from build123d import *

# Parameters (mm, degrees)
BOSS_EXTRUDE1_DEPTH  = 3.5
BOSS_EXTRUDE2_DEPTH  = 21
SKETCH3_W            = 23
SKETCH3_H            = 39
BOSS_EXTRUDE3_DEPTH  = 2.5
SKETCH5_W            = 21.5
SKETCH5_H            = 25
SKETCH5_W_2          = 7.07
SKETCH5_H_2          = 19.04
BOSS_EXTRUDE5_DEPTH  = 2.5
SKETCH6_W            = 7.07
SKETCH6_H            = 5.9
BOSS_EXTRUDE6_DEPTH  = 20
BOSS_EXTRUDE7_DEPTH  = 23
FILLET1_SIZE         = 10
SKETCH9_R            = 2.475
BOSS_EXTRUDE8_DEPTH  = 9
FILLET2_R            = 0.5
SKETCH10_R           = 1.65
CUT_EXTRUDE1_DEPTH   = 9
SKETCH11_W           = 0.2
SKETCH11_H           = 20
CUT_EXTRUDE2_DEPTH   = 9
CUT_EXTRUDE3_DEPTH   = 9
FILLET3_SIZE         = 3
BOSS_EXTRUDE9_DEPTH  = 5
SKETCH14_R           = 1.747814763
SKETCH14_R_2         = 1.6
CUT_EXTRUDE4_DEPTH   = 15
SKETCH15_W           = 110
SKETCH15_H           = 3.5
CUT_EXTRUDE5_DEPTH   = 150
FILLET4_SIZE         = 7
FILLET5_SIZE         = 3
FILLET6_SIZE         = 3
SKETCH17_W           = 8
SKETCH17_H           = 21
CUT_EXTRUDE6_DEPTH   = 150
FILLET7_R            = 1
FILLET9_SIZE         = 3
SKETCH19_R           = 1.747814763
SKETCH19_R_2         = 1.6
BOSS_EXTRUDE10_DEPTH = 8.43
CUT_EXTRUDE7_DEPTH   = 8.43
FILLET10_R           = 1


# Some blends are built 0.0001 mm under size
with BuildPart() as part:
    # Sketch1 → Boss-Extrude1 (new body)
    with BuildSketch(Plane(origin=(0, 0, 0), x_dir=(1, 0, 0), z_dir=(0, 1, 0))):
        Polygon((0, 40), (23, 40), (23, 79), (0, 79), (0, 100), (110, 100), (110, 79), (87, 79), (87, 40), (110, 40), (110, 20), (80, 0), (30, 0), (0, 20), align=None)
    extrude(amount=BOSS_EXTRUDE1_DEPTH)

    # Sketch2 → Boss-Extrude2 (add)
    with BuildSketch(Plane(origin=(0, 3.5, 0), x_dir=(1, 0, 0), z_dir=(0, 1, 0))):
        Polygon((0, 79), (23, 79), (23, 40), (0, 40), (0, 37.5), (25.5, 37.5), (25.5, 81.5), (0, 81.5), align=None)
        Polygon((110, 81.5), (84.5, 81.5), (84.5, 37.5), (110, 37.5), (110, 40), (87, 40), (87, 79), (110, 79), align=None)
    extrude(amount=BOSS_EXTRUDE2_DEPTH)

    # Sketch3 → Boss-Extrude3 (add)
    with BuildSketch(Plane(origin=(0, 24.5, 0), x_dir=(1, 0, 0), z_dir=(0, 1, 0))):
        with Locations((11.5, 59.5)):
            Rectangle(SKETCH3_W, SKETCH3_H)
        with Locations((98.5, 59.5)):
            Rectangle(SKETCH3_W, SKETCH3_H)
    extrude(amount=-BOSS_EXTRUDE3_DEPTH)

    # Sketch5 → Boss-Extrude5 (add)
    with BuildSketch(Plane(origin=(0, 24.5, 0), x_dir=(1, 0, 0), z_dir=(0, 1, 0))):
        with Locations((120.75, 50)):
            Rectangle(SKETCH5_W, SKETCH5_H)
        with Locations((-10.75, 50)):
            Rectangle(SKETCH5_W, SKETCH5_H)
        with Locations((29.035, 47.02)):
            Rectangle(SKETCH5_W_2, SKETCH5_H_2)
        with Locations((80.965, 47.02)):
            Rectangle(SKETCH5_W_2, SKETCH5_H_2)
    extrude(amount=-BOSS_EXTRUDE5_DEPTH)

    # Sketch6 → Boss-Extrude6 (add)
    with BuildSketch(Plane(origin=(0, 24.5, 0), x_dir=(1, 0, 0), z_dir=(0, 1, 0))):
        with Locations((29.035, 53.59)):
            Rectangle(SKETCH6_W, SKETCH6_H)
        with Locations((80.965, 53.59)):
            Rectangle(SKETCH6_W, SKETCH6_H)
        with Locations((-17.965, 53.59)):
            Rectangle(SKETCH6_W, SKETCH6_H)
        with Locations((127.965, 53.59)):
            Rectangle(SKETCH6_W, SKETCH6_H)
    extrude(amount=BOSS_EXTRUDE6_DEPTH)

    # Sketch7 → Boss-Extrude7 (add)
    with BuildSketch(Plane(origin=(0, 24.5, 0), x_dir=(1, 0, 0), z_dir=(0, 1, 0))):
        Polygon((0, 81.5), (25.5, 81.5), (25.5, 79), (0, 79), (-21.5, 79), (-21.5, 81.5), align=None)
        Polygon((110, 79), (84.5, 79), (84.5, 81.5), (110, 81.5), (131.5, 81.5), (131.5, 79), align=None)
    extrude(amount=BOSS_EXTRUDE7_DEPTH)

    # Fillet1
    # the kernel refuses this chamfer: 10 mm, written as the material it adds along each edge
    with BuildSketch(Plane(origin=(0, 22, -40), x_dir=(0.027495876610586372, -0.9996219169112968, 0), z_dir=(0, 0, 1)), Plane(origin=(110, 22, -37.5), x_dir=(-0.027495876610586317, -0.9996219169112968, 0), z_dir=(0, 0, -1)), Plane(origin=(110, 24.5, -81.5), x_dir=(0.9996219169112968, 0.027495876610586317, 0), z_dir=(0, 0, 1))) as fillet1_piece_1:
        Polygon((FILLET1_SIZE * 0.999621916911, -FILLET1_SIZE * 0.0274958766106), (-FILLET1_SIZE * 0.0274958766106, -FILLET1_SIZE * 0.999621916911), (0, 0), align=None)
    extrude(amount=2.5)
    with BuildSketch(Plane(origin=(0, 24.5, -79), x_dir=(0.027495876610586372, -0.9996219169112968, 0), z_dir=(0, 0, -1))) as fillet1_piece_2:
        Polygon((FILLET1_SIZE * 0.999621916911, FILLET1_SIZE * 0.0274958766106), (-FILLET1_SIZE * 0.0274958766106, FILLET1_SIZE * 0.999621916911), (0, 0), align=None)
    extrude(amount=2.5)

    # Sketch9 → Boss-Extrude8 (add)
    with BuildSketch(Plane(origin=(0, 0, -81.5), x_dir=(-1, 0, 0), z_dir=(0, 0, -1))):
        with Locations(Location((-114.55, 34.35, 0), (0, 0, 180))):
            Circle(SKETCH9_R)
        with Locations(Location((4.55, 34.35, 0), (0, 0, 180))):
            Circle(SKETCH9_R)
    extrude(amount=BOSS_EXTRUDE8_DEPTH)

    # Fillet2
    fillet2_edges = [part.edges().sort_by_distance(p)[0] for p in [
        (112.075, 34.35, -90.5),
        (-7.025, 34.35, -90.5),
    ]]
    fillet(fillet2_edges, radius=FILLET2_R)

    # Sketch10 → Cut-Extrude1 (cut)
    with BuildSketch(Plane.XY.offset(-50.64)):
        with Locations((129.16, 39.27)):
            Circle(SKETCH10_R)
        with Locations((129.16, 29.43)):
            Circle(SKETCH10_R)
        with Locations((79.77, 39.27)):
            Circle(SKETCH10_R)
        with Locations((79.77, 29.43)):
            Circle(SKETCH10_R)
        with Locations((-19.16, 29.43)):
            Circle(SKETCH10_R)
        with Locations((-19.16, 39.27)):
            Circle(SKETCH10_R)
        with Locations(Location((30.23, 39.27, 0), (0, 0, 180))):
            Circle(SKETCH10_R)
        with Locations(Location((30.23, 29.43, 0), (0, 0, 180))):
            Circle(SKETCH10_R)
    extrude(amount=-CUT_EXTRUDE1_DEPTH, mode=Mode.SUBTRACT)

    # Sketch11 → Cut-Extrude2 (cut)
    with BuildSketch(Plane.XY.offset(-50.64)):
        with Locations((-14.53, 34.5)):
            Rectangle(SKETCH11_W, SKETCH11_H)
        with Locations((25.6, 34.5)):
            Rectangle(SKETCH11_W, SKETCH11_H)
        with Locations((84.4, 34.5)):
            Rectangle(SKETCH11_W, SKETCH11_H)
        with Locations((124.53, 34.5)):
            Rectangle(SKETCH11_W, SKETCH11_H)
    extrude(amount=-CUT_EXTRUDE2_DEPTH, mode=Mode.SUBTRACT)

    # Sketch12 → Cut-Extrude3 (cut)
    with BuildSketch(Plane(origin=(0, 0, -81.5), x_dir=(-1, 0, 0), z_dir=(0, 0, -1))):
        Polygon((-108, 47.5), (-84.5, 25.5), (-84.5, 47.5), align=None)
        Polygon((-25.5, 25.5), (-25.5, 47.5), (-2, 47.5), align=None)
        Polygon((-120, 24.5), (-131.5, 36), (-131.5, 24.5), align=None)
        Polygon((10, 24.5), (21.5, 36), (21.5, 24.5), align=None)
    extrude(amount=-CUT_EXTRUDE3_DEPTH, mode=Mode.SUBTRACT)

    # Fillet3
    fillet3_edges = [part.edges().sort_by_distance(p)[0] for p in [
        (0, 23.25, -62.5),
        (110, 23.25, -62.5),
    ]]
    chamfer(fillet3_edges, length=FILLET3_SIZE)

    # Sketch13 → Boss-Extrude9 (add)
    with BuildSketch(Plane(origin=(0, 3.5, 0), x_dir=(1, 0, 0), z_dir=(0, 1, 0))):
        Polygon((0, 30.5), (32.5, 30.5), (32.5, 88.5), (0, 88.5), (0, 81.5), (25.5, 81.5), (25.5, 37.5), (0, 37.5), align=None)
        Polygon((84.5, 37.5), (110, 37.5), (110, 30.5), (77.5, 30.5), (77.5, 88.5), (110, 88.5), (110, 81.5), (84.5, 81.5), align=None)
    extrude(amount=BOSS_EXTRUDE9_DEPTH)

    # Sketch14 → Cut-Extrude4 (cut)
    with BuildSketch(Plane(origin=(0, 8.5, 0), x_dir=(1, 0, 0), z_dir=(0, 1, 0))):
        with Locations(Location((7.25, 34, 0), (0, 0, 270))):
            Circle(SKETCH14_R)
        with Locations(Location((7.25, 85, 0), (0, 0, 270))):
            Circle(SKETCH14_R_2)
        with Locations(Location((29, 34, 0), (0, 0, 270))):
            Circle(SKETCH14_R_2)
        with Locations(Location((29, 59.5, 0), (0, 0, 270))):
            Circle(SKETCH14_R_2)
        with Locations(Location((29, 85, 0), (0, 0, 270))):
            Circle(SKETCH14_R_2)
        with Locations(Location((81, 34, 0), (0, 0, 90))):
            Circle(SKETCH14_R_2)
        with Locations(Location((102.75, 34, 0), (0, 0, 90))):
            Circle(SKETCH14_R)
        with Locations(Location((81, 59.5, 0), (0, 0, 90))):
            Circle(SKETCH14_R_2)
        with Locations(Location((81, 85, 0), (0, 0, 90))):
            Circle(SKETCH14_R_2)
        with Locations(Location((102.75, 85, 0), (0, 0, 90))):
            Circle(SKETCH14_R_2)
    extrude(amount=-CUT_EXTRUDE4_DEPTH, mode=Mode.SUBTRACT)

    # Sketch15 → Cut-Extrude5 (cut)
    with BuildSketch(Plane(origin=(0, 0, -100), x_dir=(-1, 0, 0), z_dir=(0, 0, -1))):
        Polygon((-77.5, 47.5), (-77.5, 3.5), (0, 3.5), (21.5, 3.5), (21.5, 47.5), align=None)
        with Locations((-55, 1.75)):
            Rectangle(SKETCH15_W, SKETCH15_H)
    extrude(amount=-CUT_EXTRUDE5_DEPTH, mode=Mode.SUBTRACT)

    # Fillet4
    fillet4_edges = [part.edges().sort_by_distance(p)[0] for p in [
        (84.5, 22, -47.02),
    ]]
    chamfer(fillet4_edges, length=FILLET4_SIZE - 0.0001)  # a hair under: the kernel refuses the full size

    # Fillet5
    fillet5_edges = [part.edges().sort_by_distance(p)[0] for p in [
        (87, 22, -59.5),
        (98.5, 22, -79),
        (103.5, 22, -40),
    ]]
    chamfer(fillet5_edges, length=FILLET5_SIZE)

    # Fillet6
    fillet6_edges = [part.edges().sort_by_distance(p)[0] for p in [
        (110, 21.75, -79),
    ]]
    chamfer(fillet6_edges, length=FILLET6_SIZE)

    # Sketch17 → Cut-Extrude6 (cut)
    with BuildSketch(Plane.XZ.offset(-22)):
        with Locations((100, -59.5)):
            Rectangle(SKETCH17_W, SKETCH17_H)
    extrude(amount=-CUT_EXTRUDE6_DEPTH, mode=Mode.SUBTRACT)

    # Fillet7
    fillet7_edges = [part.edges().sort_by_distance(p)[0] for p in [
        (96, 23.25, -70),
        (96, 23.25, -49),
        (104, 23.25, -49),
        (104, 23.25, -70),
    ]]
    fillet(fillet7_edges, radius=FILLET7_R)

    # Fillet9
    fillet9_edges = [part.edges().sort_by_distance(p)[0] for p in [
        (87, 11.25, -79),
        (87, 11.25, -40),
    ]]
    chamfer(fillet9_edges, length=FILLET9_SIZE)

    # Sketch19 → Boss-Extrude10 (add)
    with BuildSketch(Plane.XZ.offset(-3.5)):
        Polygon((110, -40), (110, -30.5), (77.5, -30.5), (77.5, -88.5), (110, -88.5), (110, -79), (90, -79), (87, -76), (87, -43), (90, -40), align=None)
        with Locations(Location((102.75, -34, 0), (0, 0, 270))):
            Circle(SKETCH19_R, mode=Mode.SUBTRACT)
        with Locations(Location((81, -34, 0), (0, 0, 270))):
            Circle(SKETCH19_R_2, mode=Mode.SUBTRACT)
        with Locations(Location((81, -59.5, 0), (0, 0, 270))):
            Circle(SKETCH19_R_2, mode=Mode.SUBTRACT)
        with Locations(Location((81, -85, 0), (0, 0, 270))):
            Circle(SKETCH19_R_2, mode=Mode.SUBTRACT)
        with Locations(Location((102.75, -85, 0), (0, 0, 270))):
            Circle(SKETCH19_R_2, mode=Mode.SUBTRACT)
    extrude(amount=BOSS_EXTRUDE10_DEPTH)

    # Sketch20 → Cut-Extrude7 (cut)
    with BuildSketch(Plane(origin=(0, 8.5, 0), x_dir=(1, 0, 0), z_dir=(0, 1, 0))):
        Polygon((110, 88.5), (77.5, 88.5), (77.5, 81.549434768), (77.5, 30.5), (84.5, 30.5), (110, 30.5), (110, 37.5), (84.5, 37.5), (84.5, 81.549434768), (110, 81.549434768), align=None)
    extrude(amount=-CUT_EXTRUDE7_DEPTH, mode=Mode.SUBTRACT)

    # Fillet10
    fillet10_edges = [part.edges().sort_by_distance(p)[0] for p in [
        (77.5, -2.43, -30.5),
        (110, -2.43, -30.5),
        (77.5, -2.43, -88.5),
        (110, -2.43, -88.5),
    ]]
    fillet(fillet10_edges, radius=FILLET10_R)


solid = part.part
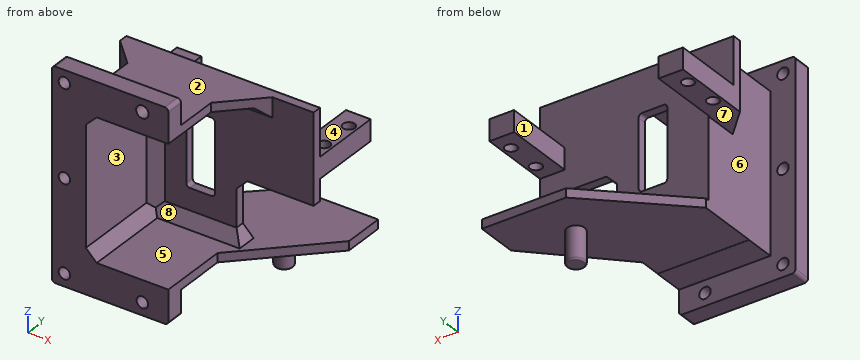
Geometry: final body of the model. Coordinates: model frame, mm. Face numbers are marked on the shaded views. A direction names the side the tool comes from. Round coordinates to 2 decimals unless told otherwise and drop trailing zeros. Loops run counter-clockwise (first coordinate to the right, second up) from the corner with the lowest first, then second, coordinate; pieces in that order, holes last. Notation, with made-up numbers: M 69,25.5 L 85,25.5 A14 ccw 85,38.5 Z; hole C 23,60 d11. An arc over 180 degrees is marked long. Put each result on its own line as item: value. Start each with the question number.
(1) Section query B-B (z = -34). Return loops of the section in (x, y).
(2) Set-up query: the marked faces 4, 5, 6, 7 and 8. Return all of +Z, -Z, +X, -X, +Y, -Y with unobstructed straight access to the full face (end or side cutting, diameter ignored); none if empty.
(3) Section query A-A (x = 126.5). Return loops of the section in (y, z).
(4) Section query C-C (z = -64.5). Return loops of the section in (x, y).
(5) Draft query along Z for the marked faces 1, 2 and 3. Return one class per face: +Z half, -Z half, draft (parallel to the pull), parting line (faces both ways), or undercut.
(6) Section query D-D (y = 39.27). Return loops of the section in (x, z), then the cut area to 3 significant figures.
(7) Material intervals for line 1 along Z through (x, y) = (81, -1.3); line 2 along Y through (x, z) = (129, -54); line 3 along X through (y, z) = (-1.75, -34), sorted ascending. Write a range as [from, to].
(8) Contact query for flat-ended pins moving along their axis: pin 1 Ø6.5 at (x, y) = (96.5, 2.5) entering from -Z; pin 2 Ø2 at (y, z) = (4.5, -76) entering from -X; pin 3 Ø3 at (y, z) = (23, -69.5) entering from +X. Output: stop coordinate, or through.
Findings below:
1. outline: M 77.5,-4.93 L 79.4,-4.93 L 79.4,0.07 L 77.5,0.07 Z; M 82.6,-4.93 L 101,-4.93 L 101,0.07 L 82.6,0.07 Z; M 104.5,-4.93 L 110,-4.93 L 110,0.07 L 104.5,0.07 Z
2. face 4: +Z, +X, -X, +Y
2. face 5: +X
2. face 6: -Z, -X
2. face 7: -Z, -X, +Y
2. face 8: +X, -Y
3. outline: M 22,-62.5 L 24.5,-62.5 L 24.5,-56.54 L 44.5,-56.54 L 44.5,-50.64 L 24.5,-50.64 L 24.5,-37.5 L 22,-37.5 Z; M 31,-81.5 L 47.5,-81.5 L 47.5,-79 L 31,-79 Z
4. outline: M 77.5,-4.93 L 87,-4.93 L 87,19 L 90,22 L 96,22 L 96,24.5 L 84.5,24.5 L 84.5,0.07 L 77.5,0.07 Z; M 104,22 L 111,22 L 111,24.5 L 104,24.5 Z
5. face 1: draft
5. face 2: +Z half
5. face 3: undercut
6. outline: M 77.5,-56.54 L 78.12,-56.54 L 78.12,-50.64 L 77.5,-50.64 Z; M 81.42,-56.54 L 84.3,-56.54 L 84.3,-50.64 L 81.42,-50.64 Z; M 99.21,-81.5 L 131.5,-81.5 L 131.5,-79 L 99.21,-79 Z; M 124.63,-56.54 L 127.51,-56.54 L 127.51,-50.64 L 124.63,-50.64 Z; M 130.81,-56.54 L 131.5,-56.54 L 131.5,-50.64 L 130.81,-50.64 Z
6. area: 122 mm2
7. line 1: z = [-88.5, -86.6], [-83.4, -61.1], [-57.9, -35.6], [-32.4, -30.5]
7. line 2: y = [22, 27.79], [31.07, 37.63], [40.91, 44.5]
7. line 3: x = [77.5, 79.4], [82.6, 101], [104.5, 110]
8. pin 1: stops at z = -88.5
8. pin 2: stops at x = 84.5
8. pin 3: stops at x = 110
